Read the model definition and answer for the solid it produces. Units are mm, in the model's axes. Face numbers are marked on the shaded views. A direction names the side the tool comes from. Round coordinates to 2 decimals unless told otherwise and drop trailing zeros. Order: outer loops, then holes, each group sorted by start corner. A loop starts at its lowest first (then second) coordinate and runs counter-clockwise, first axis right, second up. Notation, with made-up numbers: (84.5, 48) -> (135.5, 48) arc R13 ccw to (135.5, 60) -> close; hole circle Ø1 at (77.25, 13). An arc over 180 degrees is marked (long way). Use a Markdown table: item, result. Add a question column.
1. For the marked faces 1, 2 and 3, determine the directions among +Z, -Z, +X, -X, +Y, -Y from which every point of the face is accessible in a straight line to the end or side of a thin tool.
2. Consider L1, parallel to Z at x = 12.5, y = 0.5; L2, parallel to X at y = 0, z = 27; L3, parallel to Y at x = -1.5, z = 23.5. Determine where each line is inside the solid, lowest interval first. Write a range as [from, to].
3. Section B-B, the plane y = 0 is taken. Give the vertices of the cut face in (x, z).
4. Section C-C, the plane x = 0 is taken. Give the vertices of the cut face in (y, z).
5. Given pin 1 (6 mm diameter, centred on x = 22, y = 23.5, fed in from -Z); pin 2 (0.9 mm diameter, centred on y = 12, z = 17.5, fed in from +X); pin 3 (0.9 mm diameter, centred on y = -11, z = 18, fed in from +X), each flat-ended and moving along its own axis, determine where each tip first touches the part or whether it passes through.
6. Section D-D, the plane z = 20 is taken. Give the vertices of the cut face in (x, y).
7. The mould has two halves that part along Z. Classify the marked faces 4, 5, 6 and 7: +Z half, -Z half, draft (parallel to the pull), parting line (faces both ways), or undercut.
```python
from build123d import *

# Parameters (mm, degrees)
F0_W     = 66.478894
F0_H     = 91.187872
F1_DEPTH = 40
F2_R     = 11.746633
F2_R_2   = 11.746636
F3_DEPTH = 40.386
F4_R     = 9.380712
F5_DEPTH = 25.4
F6_W     = 26.066788
F6_H     = 13.062328
F7_DEPTH = 25.4
F9_DEPTH = 36.576


with BuildPart() as f1:
    # F0 (on Top) → F1 (new body)
    with BuildSketch(Plane.XY):
        Rectangle(F0_W, F0_H)
    extrude(amount=F1_DEPTH)

    # F2 (on face) → F3 (cut)
    with BuildSketch(Plane.YZ.offset(33.239447)):
        with Locations((-22.796968, 20)):
            Circle(F2_R)
        with Locations((22.796968, 20)):
            Circle(F2_R_2)
    extrude(amount=-F3_DEPTH, mode=Mode.SUBTRACT)

    # F4 (on face) → F5 (cut)
    with BuildSketch(Plane.XY.offset(40)):
        Circle(F4_R)
    extrude(amount=-F5_DEPTH, mode=Mode.SUBTRACT)

    # F6 (on face) → F7 (cut)
    with BuildSketch(Plane.YZ.offset(33.239447)):
        with Locations((0, 20)):
            Rectangle(F6_W, F6_H)
    extrude(amount=-F7_DEPTH, mode=Mode.SUBTRACT)

    # F8 (on face) → F9 (cut)
    with BuildSketch(Plane.YZ.offset(33.239447)):
        Polygon((-9.974017, 26.531164), (-9.974017, 24.998077), (-2e-06, 20), (9.974013, 24.998077), (9.974013, 26.531164), align=None)
        Polygon((-2e-06, 20), (-9.974017, 24.998077), (-9.974017, 15.001923), align=None)
        Polygon((9.974013, 24.998077), (-2e-06, 20), (9.974013, 15.001923), align=None)
        Polygon((9.974013, 15.001923), (-2e-06, 20), (-9.974017, 15.001923), (-9.974017, 13.468836), (9.974013, 13.468836), align=None)
    extrude(amount=-F9_DEPTH, mode=Mode.SUBTRACT)


solid = f1.part
```
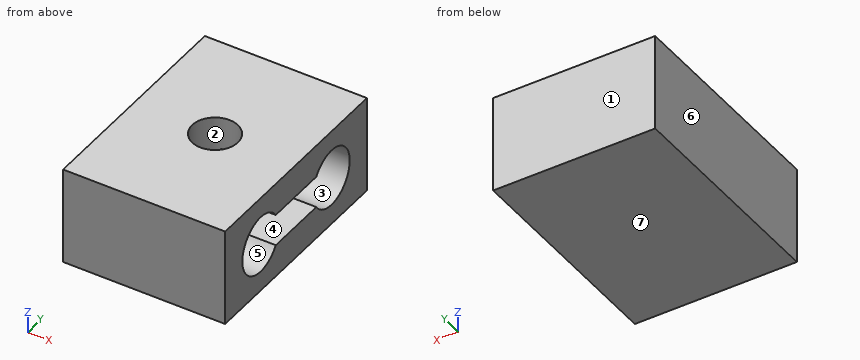
Verdict:
| question | item | result |
|---|---|---|
| 1 | face 1 | +Z, -Z, +X, -X, +Y |
| 1 | face 2 | +Z |
| 1 | face 3 | +X |
| 2 | L1 | z = [0, 13.47], [26.53, 40] |
| 2 | L2 | x = [-33.24, -9.38], [9.38, 33.24] |
| 2 | L3 | y = [-45.59, -34.01], [-11.58, -9.97], [9.97, 11.58], [34.01, 45.59] |
| 3 | outline | (-33.24, 0) -> (33.24, 0) -> (33.24, 13.47) -> (-3.34, 13.47) -> (-3.34, 14.6) -> (-9.38, 14.6) -> (-9.38, 40) -> (-33.24, 40) -> close; (9.38, 26.53) -> (33.24, 26.53) -> (33.24, 40) -> (9.38, 40) -> close |
| 4 | outline | (-45.59, 0) -> (45.59, 0) -> (45.59, 40) -> (9.38, 40) -> (9.38, 26.53) -> (9.97, 26.53) -> (9.97, 13.47) -> (-9.97, 13.47) -> (-9.97, 26.53) -> (-9.38, 26.53) -> (-9.38, 40) -> (-45.59, 40) -> close; hole circle Ø23.49 at (-22.8, 20); hole circle Ø23.49 at (22.8, 20) |
| 5 | pin 1 | stops at z = 0 |
| 5 | pin 2 | stops at x = -7.15 |
| 5 | pin 3 | stops at x = 7.84 |
| 6 | outline | (-33.24, -45.59) -> (33.24, -45.59) -> (33.24, -34.54) -> (-7.15, -34.54) -> (-7.15, -11.05) -> (7.84, -11.05) -> (7.84, -9.97) -> (-3.34, -9.97) -> (-3.34, -8.77) arc R9.38 cw to (-3.34, 8.77) -> (-3.34, 9.97) -> (7.84, 9.97) -> (7.84, 11.05) -> (-7.15, 11.05) -> (-7.15, 34.54) -> (33.24, 34.54) -> (33.24, 45.59) -> (-33.24, 45.59) -> close |
| 7 | face 4 | undercut |
| 7 | face 5 | undercut |
| 7 | face 6 | draft |
| 7 | face 7 | -Z half |
